```python
from build123d import *

# Parameters (mm, degrees)
HEAD_START           = -383.38
HEAD_CASTING_DEPTH   = 455.28
INTAKE_START         = -2.1
INTAKE_PORT_1_DEPTH  = 28
EXHAUST_START        = -4.1
EXHAUST_PORT_1_DEPTH = 32
INTAKE_START_2       = -113.86
INTAKE_PORT_3_DEPTH  = 28
EXHAUST_START_2      = -115.86
EXHAUST_PORT_3_DEPTH = 32
INTAKE_START_3       = -225.62
INTAKE_PORT_5_DEPTH  = 28
EXHAUST_START_3      = -227.62
EXHAUST_PORT_5_DEPTH = 32
INTAKE_START_4       = -337.38
INTAKE_PORT_7_DEPTH  = 28
EXHAUST_START_4      = -339.38
EXHAUST_PORT_7_DEPTH = 32


with BuildPart() as part:
    # Sketch1 → Head Casting (new body)
    with BuildSketch(Plane.XY.offset(HEAD_START)):
        with BuildLine():
            Line((115.223049994, 217.046426485), (217.046426485, 115.223049994))
            Line((217.046426485, 115.223049994), (287.757104604, 185.933728113))
            ThreePointArc((287.757104604, 185.933728113), (289.221570698, 189.469262019), (287.757104604, 193.004795925))
            Line((287.757104604, 193.004795925), (193.004795925, 287.757104604))
            ThreePointArc((193.004795925, 287.757104604), (189.469262019, 289.221570698), (185.933728113, 287.757104604))
            Line((185.933728113, 287.757104604), (115.223049994, 217.046426485))
        make_face()
    extrude(amount=HEAD_CASTING_DEPTH)

    # Sketch2 → Intake Port 1 (cut)
    with BuildSketch(Plane.XY.offset(INTAKE_START)):
        with BuildLine():
            Line((135.729146649, 238.966736702), (153.406816178, 221.289067172))
            ThreePointArc((153.406816178, 221.289067172), (157.649456866, 219.531707859), (161.892097553, 221.289067172))
            Line((161.892097553, 221.289067172), (181.691087426, 241.088057046))
            ThreePointArc((181.691087426, 241.088057046), (183.448446739, 245.330697733), (181.691087426, 249.57333842))
            Line((181.691087426, 249.57333842), (164.013417896, 267.251007949))
            Line((164.013417896, 267.251007949), (135.729146649, 238.966736702))
        make_face()
    extrude(amount=INTAKE_PORT_1_DEPTH, mode=Mode.SUBTRACT)

    # Sketch3 → Exhaust Port 1 (cut)
    with BuildSketch(Plane.XY.offset(EXHAUST_START)):
        with BuildLine():
            Line((240.380950264, 137.143360211), (224.117494297, 153.406816178))
            ThreePointArc((224.117494297, 153.406816178), (221.774348547, 159.063670428), (224.117494297, 164.720524677))
            Line((224.117494297, 164.720524677), (238.259629921, 178.862660301))
            ThreePointArc((238.259629921, 178.862660301), (243.91648417, 181.205806052), (249.57333842, 178.862660301))
            Line((249.57333842, 178.862660301), (265.836794387, 162.599204334))
            Line((265.836794387, 162.599204334), (240.380950264, 137.143360211))
        make_face()
    extrude(amount=EXHAUST_PORT_1_DEPTH, mode=Mode.SUBTRACT)

    # Sketch4 → Intake Port 3 (cut)
    with BuildSketch(Plane.XY.offset(INTAKE_START_2)):
        with BuildLine():
            Line((135.729146649, 238.966736702), (153.406816178, 221.289067172))
            ThreePointArc((153.406816178, 221.289067172), (157.649456866, 219.531707859), (161.892097553, 221.289067172))
            Line((161.892097553, 221.289067172), (181.691087426, 241.088057046))
            ThreePointArc((181.691087426, 241.088057046), (183.448446739, 245.330697733), (181.691087426, 249.57333842))
            Line((181.691087426, 249.57333842), (164.013417896, 267.251007949))
            Line((164.013417896, 267.251007949), (135.729146649, 238.966736702))
        make_face()
    extrude(amount=INTAKE_PORT_3_DEPTH, mode=Mode.SUBTRACT)

    # Sketch5 → Exhaust Port 3 (cut)
    with BuildSketch(Plane.XY.offset(EXHAUST_START_2)):
        with BuildLine():
            Line((240.380950264, 137.143360211), (224.117494297, 153.406816178))
            ThreePointArc((224.117494297, 153.406816178), (221.774348547, 159.063670428), (224.117494297, 164.720524677))
            Line((224.117494297, 164.720524677), (238.259629921, 178.862660301))
            ThreePointArc((238.259629921, 178.862660301), (243.91648417, 181.205806052), (249.57333842, 178.862660301))
            Line((249.57333842, 178.862660301), (265.836794387, 162.599204334))
            Line((265.836794387, 162.599204334), (240.380950264, 137.143360211))
        make_face()
    extrude(amount=EXHAUST_PORT_3_DEPTH, mode=Mode.SUBTRACT)

    # Sketch6 → Intake Port 5 (cut)
    with BuildSketch(Plane.XY.offset(INTAKE_START_3)):
        with BuildLine():
            Line((135.729146649, 238.966736702), (153.406816178, 221.289067172))
            ThreePointArc((153.406816178, 221.289067172), (157.649456866, 219.531707859), (161.892097553, 221.289067172))
            Line((161.892097553, 221.289067172), (181.691087426, 241.088057046))
            ThreePointArc((181.691087426, 241.088057046), (183.448446739, 245.330697733), (181.691087426, 249.57333842))
            Line((181.691087426, 249.57333842), (164.013417896, 267.251007949))
            Line((164.013417896, 267.251007949), (135.729146649, 238.966736702))
        make_face()
    extrude(amount=INTAKE_PORT_5_DEPTH, mode=Mode.SUBTRACT)

    # Sketch7 → Exhaust Port 5 (cut)
    with BuildSketch(Plane.XY.offset(EXHAUST_START_3)):
        with BuildLine():
            Line((240.380950264, 137.143360211), (224.117494297, 153.406816178))
            ThreePointArc((224.117494297, 153.406816178), (221.774348547, 159.063670428), (224.117494297, 164.720524677))
            Line((224.117494297, 164.720524677), (238.259629921, 178.862660301))
            ThreePointArc((238.259629921, 178.862660301), (243.91648417, 181.205806052), (249.57333842, 178.862660301))
            Line((249.57333842, 178.862660301), (265.836794387, 162.599204334))
            Line((265.836794387, 162.599204334), (240.380950264, 137.143360211))
        make_face()
    extrude(amount=EXHAUST_PORT_5_DEPTH, mode=Mode.SUBTRACT)

    # Sketch8 → Intake Port 7 (cut)
    with BuildSketch(Plane.XY.offset(INTAKE_START_4)):
        with BuildLine():
            Line((135.729146649, 238.966736702), (153.406816178, 221.289067172))
            ThreePointArc((153.406816178, 221.289067172), (157.649456866, 219.531707859), (161.892097553, 221.289067172))
            Line((161.892097553, 221.289067172), (181.691087426, 241.088057046))
            ThreePointArc((181.691087426, 241.088057046), (183.448446739, 245.330697733), (181.691087426, 249.57333842))
            Line((181.691087426, 249.57333842), (164.013417896, 267.251007949))
            Line((164.013417896, 267.251007949), (135.729146649, 238.966736702))
        make_face()
    extrude(amount=INTAKE_PORT_7_DEPTH, mode=Mode.SUBTRACT)

    # Sketch9 → Exhaust Port 7 (cut)
    with BuildSketch(Plane.XY.offset(EXHAUST_START_4)):
        with BuildLine():
            Line((240.380950264, 137.143360211), (224.117494297, 153.406816178))
            ThreePointArc((224.117494297, 153.406816178), (221.774348547, 159.063670428), (224.117494297, 164.720524677))
            Line((224.117494297, 164.720524677), (238.259629921, 178.862660301))
            ThreePointArc((238.259629921, 178.862660301), (243.91648417, 181.205806052), (249.57333842, 178.862660301))
            Line((249.57333842, 178.862660301), (265.836794387, 162.599204334))
            Line((265.836794387, 162.599204334), (240.380950264, 137.143360211))
        make_face()
    extrude(amount=EXHAUST_PORT_7_DEPTH, mode=Mode.SUBTRACT)


solid = part.part
```
Geometry: final body of the model. Coordinates: model frame, mm. A direction names the side the tool comes from. Give positions to 0.01 mm unless a question says otherwise; leave off trailing zeros. Loops run counter-clockwise (first coordinate to the right, second up) from the corner with the lowest first, then second, coordinate; pieces in that order, holes last. Notation, with made-up numbers: (39, -21) -> (89, -21) arc R16 ccw to (89, -5) -> close; hole circle Ø5 at (0, 78.5). An arc over 180 degrees is marked (long way). Return JSON: item names as keys, results as strings.
Item 1: Line query: line 1 (Z direction, x = 232, y = 152); line 2 (Y direction, x = 178, z = -211.5); line 3 (Y direction, x = 227, z = -222.5). Output: solid intervals per line, ascending.
Filled in:
{"line 1": "-383.38 to -339.38, -307.38 to -227.62, -195.62 to -115.86, -83.86 to -4.1, 27.9 to 71.9", "line 2": "154.27 to 237.4, 253.26 to 279.82", "line 3": "125.18 to 150.52, 167.6 to 253.76"}
Item 2: Pin query (flat end, axial travel): P1, Ø8, axis at x = 193, z = -188, coming from the -Y side; P2, Ø6, axis at x = 230.5, z = -173.5, coming from the +Y side; P3, Ø8, axis at y = 147, z = -240.5, coming from the -X side. Return the tip coordinate at first contact, or that it passes through.
Filled in:
{"P1": "y = 135.27", "P2": "y = 253.26", "P3": "x = 181.27"}
Item 3: Section B-B, the plane z = -249.5. Output: boundary loops of the cut face in (x, y), plus the area to 3 significant figures.
Filled in:
{"outline": "(115.22, 217.05) -> (217.05, 115.22) -> (287.76, 185.93) arc R5 ccw to (287.76, 193) -> (193, 287.76) arc R5 ccw to (185.93, 287.76) -> close", "area": "15,100 mm^2"}
Item 4: Section C-C, the plane x = 274. Output: boundary loops of the cut face in (y, z), plus the area to 3 significant figures.
Filled in:
{"outline": "(172.18, -383.38) -> (206.76, -383.38) -> (206.76, 71.9) -> (172.18, 71.9) -> close", "area": "15,700 mm^2"}
Item 5: Access query for faces 1 (the flat face through (144.803, 229.893, 11.704)), 2 (the flat face through (232.005, 145.52, -211.844)), 3 (the flat face through (160, 243, -85.86)), 4 (the cylindrical face through (183.45, 245.26, -100.06)). Directions: +Z, -Z, +X, -X, +Y, -Y. A direction counts if a zero-diameter tool reaches every point of the face in a straight line with its end or side. Return the directions, or none.
Filled in:
{"face 1": "+Y", "face 2": "+X", "face 3": "none", "face 4": "-X"}
Item 6: Mould query, pull axis Y, two halves, no side actions, for faces 5 (the flat face through (151.073, 252.897, -158.927)), 6 (the flat face through (165.42, 166.85, -158.93)), 7 (the flat face through (171.653, 231.05, 11.704)). Classes: released by +Y, released by -Y, zero draft, split by the parting line, or undercut.
Filled in:
{"face 5": "released by +Y", "face 6": "released by -Y", "face 7": "undercut"}
Item 7: Section D-D, the plane y = 273. Output: boundary loops of the cut face in (x, z), plus the area to 3 significant figures.
Filled in:
{"outline": "(171.18, -383.38) -> (207.76, -383.38) -> (207.76, 71.9) -> (171.18, 71.9) -> close", "area": "16,700 mm^2"}
Item 8: Section A-A, the plane x = 233. Output: boundary loops of the cut face in (y, z).
Filled in:
{"outline": "(131.18, -383.38) -> (247.76, -383.38) -> (247.76, 71.9) -> (131.18, 71.9) -> close; hole (144.52, -339.38) -> (173.6, -339.38) -> (173.6, -307.38) -> (144.52, -307.38) -> close; hole (144.52, -227.62) -> (173.6, -227.62) -> (173.6, -195.62) -> (144.52, -195.62) -> close; hole (144.52, -115.86) -> (173.6, -115.86) -> (173.6, -83.86) -> (144.52, -83.86) -> close; hole (144.52, -4.1) -> (173.6, -4.1) -> (173.6, 27.9) -> (144.52, 27.9) -> close"}
